from build123d import *

# Parameters (mm, degrees)
SKETCH1_W                    = 40
SKETCH1_H                    = 30
BOSS_EXTRUDE1_DEPTH          = 10
SKETCH2_W                    = 28
SKETCH2_H                    = 18
CUT_EXTRUDE1_DEPTH           = 43.801869118
CUT_EXTRUDE2_DEPTH           = 2
CUT_EXTRUDE3_DEPTH           = 2
CUT_EXTRUDE4_DEPTH           = 2
CUT_EXTRUDE5_DEPTH           = 2
F_3_0_3_DIAMETER_HOLE1_D     = 3
F_3_0_3_DIAMETER_HOLE1_DEPTH = 4
F_3_0_3_DIAMETER_HOLE2_D     = 3
F_3_0_3_DIAMETER_HOLE2_DEPTH = 4
F_3_0_3_DIAMETER_HOLE3_D     = 3
F_3_0_3_DIAMETER_HOLE4_D     = 3


with BuildPart() as part:
    # Sketch1 → Boss-Extrude1 (new body)
    with BuildSketch(Plane(origin=(0, 0, 0), x_dir=(-1, 0, 0), z_dir=(0, 0, -1))):
        with Locations((-14, 9)):
            Rectangle(SKETCH1_W, SKETCH1_H)
    extrude(amount=-BOSS_EXTRUDE1_DEPTH)

    # Sketch2 → Cut-Extrude1 (cut, through all)
    with BuildSketch(Plane.XY.offset(10)):
        with Locations((14, 9)):
            Rectangle(SKETCH2_W, SKETCH2_H)
    extrude(amount=-CUT_EXTRUDE1_DEPTH, mode=Mode.SUBTRACT)

    # Sketch3 → Cut-Extrude2 (cut)
    with BuildSketch(Plane(origin=(0, 0, 0), x_dir=(0, 0, -1), z_dir=(1, 0, 0))):
        Polygon((-8.25, 9), (-6.625, 6.185417438), (-3.375, 6.185417438), (-1.75, 9), (-3.375, 11.814582562), (-6.625, 11.814582562), align=None)
    extrude(amount=-CUT_EXTRUDE2_DEPTH, mode=Mode.SUBTRACT)

    # Sketch4 → Cut-Extrude3 (cut)
    with BuildSketch(Plane.XZ.offset(-18)):
        Polygon((17.25, 5), (15.625, 7.814582562), (12.375, 7.814582562), (10.75, 5), (12.375, 2.185417438), (15.625, 2.185417438), align=None)
    extrude(amount=-CUT_EXTRUDE3_DEPTH, mode=Mode.SUBTRACT)

    # Sketch5 → Cut-Extrude4 (cut)
    with BuildSketch(Plane.ZY.offset(-28)):
        Polygon((1.75, 9), (3.375, 6.185417438), (6.625, 6.185417438), (8.25, 9), (6.625, 11.814582562), (3.375, 11.814582562), align=None)
    extrude(amount=-CUT_EXTRUDE4_DEPTH, mode=Mode.SUBTRACT)

    # Sketch6 → Cut-Extrude5 (cut)
    with BuildSketch(Plane(origin=(0, 0, 0), x_dir=(-1, 0, 0), z_dir=(0, 1, 0))):
        Polygon((-17.25, 5), (-15.625, 2.185417438), (-12.375, 2.185417438), (-10.75, 5), (-12.375, 7.814582562), (-15.625, 7.814582562), align=None)
    extrude(amount=-CUT_EXTRUDE5_DEPTH, mode=Mode.SUBTRACT)

    # Ø3.0 (3) Diameter Hole1
    with Locations(Plane(origin=(-2, 0, 0), x_dir=(0, 0, -1), z_dir=(1, 0, 0))):
        with Locations((-5, 9)):
            Hole(F_3_0_3_DIAMETER_HOLE1_D / 2, depth=F_3_0_3_DIAMETER_HOLE1_DEPTH)

    # Ø3.0 (3) Diameter Hole2
    with Locations(Plane(origin=(0, 20, 0), x_dir=(-1, 0, 0), z_dir=(0, -1, 0))):
        with Locations((-14, -5)):
            Hole(F_3_0_3_DIAMETER_HOLE2_D / 2, depth=F_3_0_3_DIAMETER_HOLE2_DEPTH)

    # Ø3.0 (3) Diameter Hole3 (through all)
    with Locations(Plane.ZY.offset(-30)):
        with Locations((5, 9)):
            Hole(F_3_0_3_DIAMETER_HOLE3_D / 2)

    # Ø3.0 (3) Diameter Hole4 (through all)
    with Locations(Plane(origin=(0, -2, 0), x_dir=(1, 0, 0), z_dir=(0, 1, 0))):
        with Locations((14, -5)):
            Hole(F_3_0_3_DIAMETER_HOLE4_D / 2)


solid = part.part
For this review, take the finished solid that the model builds, in its own axes (mm). A direction names the side the tool comes from. Round coordinates to 2 decimals unless told otherwise and drop trailing zeros. Loops run counter-clockwise (first coordinate to the right, second up) from the corner with the lowest first, then second, coordinate; pieces in that order, holes last. Notation, with made-up numbers: (-40, -5.5) - (-36, -5.5) arc R32 cw to (-36, 23.5) - close; hole circle Ø8 at (-13, -17.5). An arc over 180 degrees is marked (long way). Use one line per item in the form item = value.
1) Tool access review of faces 4 (the face through (14, 19, 0)), 5 (the face through (28.986, 10.388, 7.449)), 6 (the face through (11, 18, 6)): name each direction out of +Z, -Z, +X, -X, +Y, -Y from which nothing blocks a thin tool from reaching the whole face with its end or side.
Solutions:
face_4 = -Z, +X, -X, +Y, -Y
face_5 = none
face_6 = +Z, -Z
2) We need section D-D on x = 18.5. Write out the cut boundary in (y, z), then the cut area to 3 significant figures.
Solutions:
outline = (-6, 0) - (0, 0) - (0, 10) - (-6, 10) - close; (18, 0) - (24, 0) - (24, 10) - (18, 10) - close
area = 120 mm2
3) We need section C-C on y = 5. Write out the cut boundary in (x, z).
Solutions:
outline = (-6, 0) - (0, 0) - (0, 10) - (-6, 10) - close; (28, 0) - (34, 0) - (34, 10) - (28, 10) - close
4) Wall thickness on probe 1 along Y at (x, z) = (16.5, 0.5); probe 2 along X at (y, z) = (8, 2.25); probe 3 along X at (y, z) = (9, 2.75): over which ranges is each line inside the solid? List them lowest first.
Solutions:
probe_1 = -6 to 0, 18 to 24
probe_2 = -6 to 0, 28 to 34
probe_3 = -6 to -2, 30 to 34
5) Clearance check with a flat-ended pin moving along its axis: P1, Ø10, axis at x = 20.5, y = 12, coming from the +Z side. State where the tip first meets the part, or that it passes through.
Solutions:
P1 = through
6) Mouldability with a two-part tool opening along X and no side actions: class faces 1 (the face through (14, -6, 3)), 2 (the face through (14, -1, 2.185)), 3 (the face through (34, 9, 3)) as pulls with the +X half, pulls with the -X half, needs draft (parallel to the pull), parting line crosses it, or undercut.
Solutions:
face_1 = needs draft
face_2 = undercut
face_3 = pulls with the +X half
7) We need section B-B on x = 14. Write out the cut boundary in (y, z).
Solutions:
outline = (-6, 0) - (0, 0) - (0, 2.19) - (-2, 2.19) - (-2, 3.5) - (-6, 3.5) - close; (-6, 6.5) - (-2, 6.5) - (-2, 7.81) - (0, 7.81) - (0, 10) - (-6, 10) - close; (18, 0) - (24, 0) - (24, 3.5) - (20, 3.5) - (20, 2.19) - (18, 2.19) - close; (18, 7.81) - (20, 7.81) - (20, 6.5) - (24, 6.5) - (24, 10) - (18, 10) - close
8) We need section A-A on y = -1. Write out the cut boundary in (x, z) (3 decimals).
Solutions:
outline = (-6, 0) - (34, 0) - (34, 10) - (-6, 10) - close; hole (10.75, 5) - (12.375, 2.185) - (15.625, 2.185) - (17.25, 5) - (15.625, 7.815) - (12.375, 7.815) - close
